The model under review builds one solid part; all positions refer to its coordinate system, in mm. A direction names the side the tool comes from. Round coordinates to 2 decimals unless told otherwise and drop trailing zeros. Write each loop counter-clockwise with the first axis right and the second up, starting at its lowest first coordinate (ties: lowest second). Pieces come first, ordered by that corner, then holes. Notation, with made-up numbers: (-4, 67) - (49, 67) arc R25 ccw to (49, 102) - close; hole circle Ø2 at (74, 21.25). An arc over 180 degrees is marked (long way). Write each question's results on one line, items separated by ' | '.
```python
from build123d import *

# Parameters (mm, degrees)
SKETCH_1_W      = 62
SKETCH_1_H      = 40
SKETCH_1_R      = 2.25
EXTRUDE_1_DEPTH = 2.5
SKETCH_2_W      = 46.5
SKETCH_2_H      = 42.7
SKETCH_2_R      = 11.525
SKETCH_2_R_2    = 1.75
EXTRUDE_2_DEPTH = 2.2
EXTRUDE_3_DEPTH = 1.6
EXTRUDE_4_DEPTH = 1.6


with BuildPart() as part:
    # Эскиз1 → Бобышка-Вытянуть1 (new body)
    with BuildSketch(Plane(origin=(0, 0, 0), x_dir=(1, 0, 0), z_dir=(0, 1, 0))):
        Rectangle(SKETCH_1_W, SKETCH_1_H)
        with Locations(Location((-27, 0, 0), (0, 0, 270))):
            Circle(SKETCH_1_R, mode=Mode.SUBTRACT)
        with Locations(Location((27, 0, 0), (0, 0, 270))):
            Circle(SKETCH_1_R, mode=Mode.SUBTRACT)
        with Locations(Location((-27, 15, 0), (0, 0, 270))):
            Circle(SKETCH_1_R, mode=Mode.SUBTRACT)
        with Locations(Location((27, 15, 0), (0, 0, 270))):
            Circle(SKETCH_1_R, mode=Mode.SUBTRACT)
        with Locations(Location((-27, -15, 0), (0, 0, 270))):
            Circle(SKETCH_1_R, mode=Mode.SUBTRACT)
        with Locations(Location((27, -15, 0), (0, 0, 270))):
            Circle(SKETCH_1_R, mode=Mode.SUBTRACT)
    extrude(amount=EXTRUDE_1_DEPTH)

    # Эскиз2 → Бобышка-Вытянуть2 (add)
    with BuildSketch(Plane.XY.offset(20)):
        with Locations((0, 23.85)):
            Rectangle(SKETCH_2_W, SKETCH_2_H)
        with Locations((0, 23.875)):
            Circle(SKETCH_2_R, mode=Mode.SUBTRACT)
        with Locations((15.5, 39.375)):
            Circle(SKETCH_2_R_2, mode=Mode.SUBTRACT)
        with Locations((15.5, 8.375)):
            Circle(SKETCH_2_R_2, mode=Mode.SUBTRACT)
        with Locations((-15.5, 8.375)):
            Circle(SKETCH_2_R_2, mode=Mode.SUBTRACT)
        with Locations((-15.5, 39.375)):
            Circle(SKETCH_2_R_2, mode=Mode.SUBTRACT)
    extrude(amount=-EXTRUDE_2_DEPTH)

    # Эскиз3 → Бобышка-Вытянуть3 (add)
    with BuildSketch(Plane.ZY.offset(23.25)):
        Polygon((-20, 2.5), (17.8, 45.2), (17.8, 2.5), align=None)
    extrude(amount=-EXTRUDE_3_DEPTH)

    # Эскиз4 → Бобышка-Вытянуть4 (add)
    with BuildSketch(Plane(origin=(23.25, 0, 0), x_dir=(0, 0, -1), z_dir=(1, 0, 0))):
        Polygon((-17.8, 2.5), (20, 2.5), (-17.8, 45.2), align=None)
    extrude(amount=-EXTRUDE_4_DEPTH)


solid = part.part
```
Q1. We need section A-A (x = 15.5). State the section outline as (y, z) points (3 decimals).
Evaluation:
outline: (0, -20) - (2.5, -20) - (2.5, 17.8) - (6.625, 17.8) - (6.625, 20) - (0, 20) - close; (10.125, 17.8) - (37.625, 17.8) - (37.625, 20) - (10.125, 20) - close; (41.125, 17.8) - (45.2, 17.8) - (45.2, 20) - (41.125, 20) - close
Q2. For probe 1 along Y at (x, z) = (15.5, 19.45) (3 decimals); probe 2 along X at (y, z) = (0.8, 15); probe 3 along X at (y, z) = (16.5, 1), list the stretches that pass through material, from the lowest coordinate up.
Evaluation:
probe 1: y = 0 to 6.625, 10.125 to 37.625, 41.125 to 45.2 | probe 2: x = -31 to -29.25, -24.75 to 24.75, 29.25 to 31 | probe 3: x = -23.25 to -21.65, 21.65 to 23.25
Q3. Tool access review of faces 5 (the flat face through (21.65, 15, 8)), 6 (the flat face through (0, 1, -20)): name each direction out of +Z, -Z, +X, -X, +Y, -Y from which nothing blocks a thin tool from reaching the whole face with its end or side.
Evaluation:
face 5: -Z, +Y | face 6: -Z, +X, -X, +Y, -Y
Q4. We need section D-D (x = -3). State the section outline as (y, z) points, plus the area to 3 significant figures.
Evaluation:
outline: (0, -20) - (2.5, -20) - (2.5, 17.8) - (12.75, 17.8) - (12.75, 20) - (0, 20) - close; (35, 17.8) - (45.2, 17.8) - (45.2, 20) - (35, 20) - close | area: 145 mm^2
Q5. The part is to be moulded in two halves that separate along X. For faces 1 (the flat face through (31, 1, 0)), 2 (the cylindrical face through (-13.83, 8.9, 18.92)), 3 (the flat face through (30, 2.5, 0)), 4 (the cylindrical face through (-29.196, 1.232, -0.488)), say which applies: released by +X, released by -X, zero draft, split by the parting line, or undercut.
Evaluation:
face 1: released by +X | face 2: undercut | face 3: zero draft | face 4: undercut
Q6. We need section C-C (z = 15). State the section outline as (x, y) points, plus the area to 3 significant figures.
Evaluation:
outline: (-31, 0) - (-29.25, 0) - (-29.25, 2.5) - (-31, 2.5) - close; (-24.75, 0) - (24.75, 0) - (24.75, 2.5) - (23.25, 2.5) - (23.25, 42.04) - (21.65, 42.04) - (21.65, 2.5) - (-21.65, 2.5) - (-21.65, 42.04) - (-23.25, 42.04) - (-23.25, 2.5) - (-24.75, 2.5) - close; (29.25, 0) - (31, 0) - (31, 2.5) - (29.25, 2.5) - close | area: 259 mm^2
Q7. Insertion check: P1, Ø8, axis at x = -14, y = 31.5, coming from the -Z side; P2, Ø2.5, axis at x = -26, z = -5.5, coming from the +Y side; P3, Ø4, axis at x = -22.5, z = -3, coming from the +Y side. Each pin has a flat end and moves straight along its axis. Give the tip position at first contact, or say it passes through.
Evaluation:
P1: stops at z = 17.8 | P2: stops at y = 2.5 | P3: stops at y = 23.96
Q8. We need section B-B (y = 22). State the section outline as (x, z) points.
Evaluation:
outline: (-23.25, -2.74) - (-21.65, -2.74) - (-21.65, 17.8) - (-11.37, 17.8) - (-11.37, 20) - (-23.25, 20) - close; (11.37, 17.8) - (21.65, 17.8) - (21.65, -2.74) - (23.25, -2.74) - (23.25, 20) - (11.37, 20) - close
